The listing builds one solid part. Answer for the finished solid, in the listing's coordinates (mm). A direction names the side the tool comes from. Coordinates: 2 decimals unless noted, no trailing zeros. Write each loop counter-clockwise with the first axis right and the second up, starting at its lowest first coordinate (ties: lowest second). Pieces come first, ordered by that corner, then holes.
from build123d import *

# Parameters (mm, degrees)
SKETCH_W        = 130
SKETCH_H        = 90
PAD_DEPTH       = 5
CHAMFER_SIZE    = 30
SKETCH001_W     = 19.5
SKETCH001_H     = 22.5
POCKET_DEPTH    = 5
SKETCH002_W     = 7
SKETCH002_H     = 10
POCKET001_DEPTH = 5


with BuildPart() as part:
    # Sketch → Pad (new body)
    with BuildSketch(Plane.XY):
        Rectangle(SKETCH_W, SKETCH_H)
    extrude(amount=PAD_DEPTH)

    # Chamfer
    chamfer_edges = [part.edges().sort_by_distance(p)[0] for p in [
        (-65, -45, 2.5),
        (65, -45, 2.5),
        (65, 45, 2.5),
        (-65, 45, 2.5),
    ]]
    chamfer(chamfer_edges, length=CHAMFER_SIZE)

    # Sketch001 (on Face5 of Chamfer) → Pocket (cut)
    with BuildSketch(Plane.XY.offset(5)):
        with Locations((55.25, 0)):
            Rectangle(SKETCH001_W, SKETCH001_H)
        with Locations((-55.25, 0)):
            Rectangle(SKETCH001_W, SKETCH001_H)
    extrude(amount=-POCKET_DEPTH, mode=Mode.SUBTRACT)

    # Sketch002 (on Face5 of Pocket) → Pocket001 (cut)
    with BuildSketch(Plane.XY.offset(5)):
        with Locations((46, -20.744505)):
            Rectangle(SKETCH002_W, SKETCH002_H)
    extrude(amount=-POCKET001_DEPTH, mode=Mode.SUBTRACT)


solid = part.part
Q1. Find the intervals of material crossed by probe 1 along X at (y, z) = (8, 4.7); probe 2 along Y at (x, z) = (-46, 0.9); probe 3 along X at (y, z) = (38, 3.2), in increasing order.
Answers below:
probe 1: x = -45.5 to 45.5
probe 2: y = -34 to -11.25, 11.25 to 34
probe 3: x = -42 to 42
Q2. Given pin 1 (2.5 mm diameter, centred on x = -59.5, z = 3.5, fed in from -Y); pin 2 (3 mm diameter, centred on x = -48, z = 4, fed in from +Y); pin 3 (2.5 mm diameter, centred on y = -23, z = 3.5, fed in from -X), each flat-ended and moving along its own axis, determine where each tip first touches the part or whether it passes through.
Answers below:
pin 1: stops at y = -21.75
pin 2: stops at y = 33.5
pin 3: stops at x = -58.25
Q3. Determine the mould class of faces 1 (the face through (46, -25.745, 3)), 2 (the face through (-45.5, 0, 3)), 3 (the face through (50, 30, 2)), 4 (the face through (-55, 11.25, 3)) for opening direction X: released by +X, released by -X, zero draft, split by the parting line, or undercut.
Answers below:
face 1: undercut
face 2: released by -X
face 3: released by +X
face 4: zero draft
Q4. The part is cut by section D-D, the plane x = 40. Write down the section's boundary in (y, z).
Answers below:
outline: (-40, 0) - (40, 0) - (40, 5) - (-40, 5) - close
Q5. The part is cut by section C-C, the plane y = 20. Write down the section's boundary in (x, z).
Answers below:
outline: (-60, 0) - (60, 0) - (60, 5) - (-60, 5) - close
Q6. The part is cut by section A-A, the plane z = 4.25. Write down the section's boundary in (x, y).
Answers below:
outline: (-65, -15) - (-35, -45) - (35, -45) - (65, -15) - (65, -11.25) - (45.5, -11.25) - (45.5, 11.25) - (65, 11.25) - (65, 15) - (35, 45) - (-35, 45) - (-65, 15) - (-65, 11.25) - (-45.5, 11.25) - (-45.5, -11.25) - (-65, -11.25) - close; hole (42.5, -25.74) - (49.5, -25.74) - (49.5, -15.74) - (42.5, -15.74) - close
Q7. The part is cut by section B-B, the plane x = -53.5. Write down the section's boundary in (y, z), then the cut area to 4 significant figures.
Answers below:
outline: (-26.5, 0) - (-11.25, 0) - (-11.25, 5) - (-26.5, 5) - close; (11.25, 0) - (26.5, 0) - (26.5, 5) - (11.25, 5) - close
area: 152.5 mm2
Q8. Which of the six approach directions +Z, -Z, +X, -X, +Y, -Y give full straight-line access (tool end or side, diameter ignored) to faces 5 (the face through (45.5, 0, 3)), 6 (the face through (0, -45, 2)), 7 (the face through (46, -15.745, 3))?
Answers below:
face 5: +Z, -Z, +X
face 6: +Z, -Z, +X, -X, -Y
face 7: +Z, -Z
